Check sheet for the drawn part. Datum: minimum x, y, z corner. Units: mm. Round coordinates to 2 decimals unless told otherwise and drop trailing zeros. Order: outer loops, then holes, each group sorted by start corner. A loop starts at its lowest first (then second) coordinate and runs counter-clockwise, first axis right, second up. Notation, with made-up numbers: M -39,49 L 14,49 A10 cw 14,62 Z; hole C 16.5,-23 d11. An arc over 180 degrees is marked long. Write item = value, one per line. Start each with the question number.
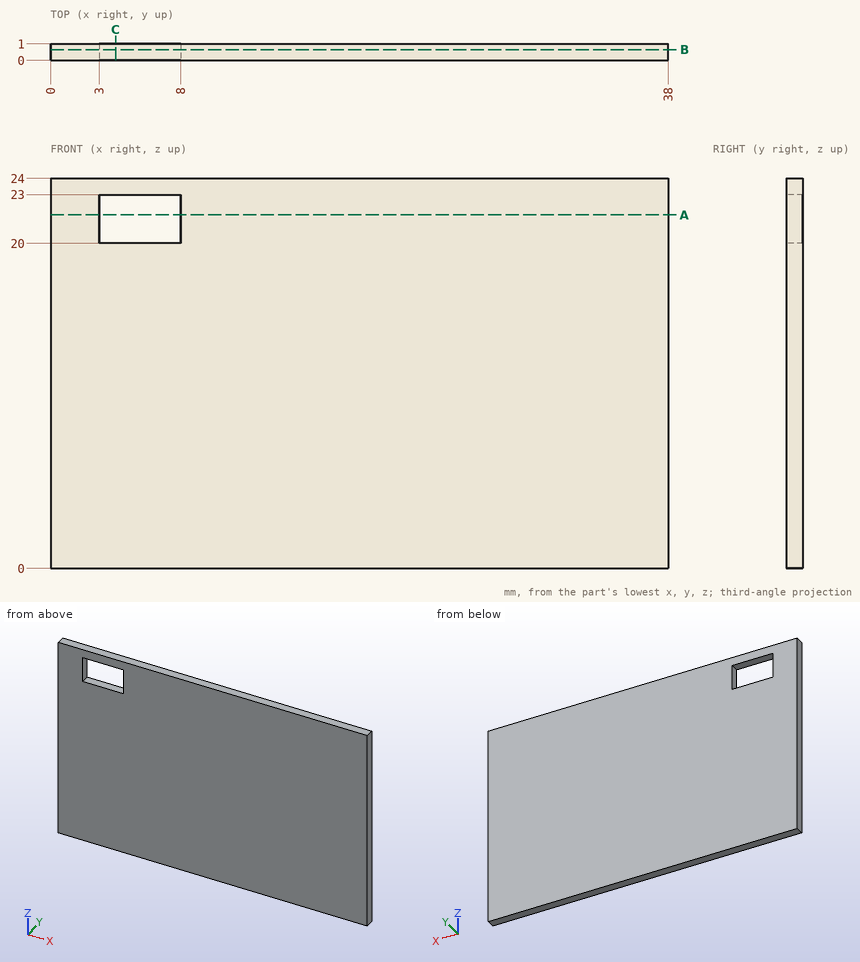
1) Cross-section at A-A, the plane z = 21.75. Enter the section's corners in (x, y).
2) Cross-section at B-B, the plane y = 0.65. Enter the section's corners in (x, z).
3) Cross-section at C-C, the plane x = 4. Enter the section's corners in (y, z), then the cut area to 3 significant figures.
4) Scan lines: probe 1 along X at (y, z) = (0.75, 20.25); probe 2 along Z at (x, y) = (4, 0.3). Record each from-to range of solid material in increasing order.
Geometry results:
q1.outline = M 0,0 L 3,0 L 3,1 L 0,1 Z; M 8,0 L 38,0 L 38,1 L 8,1 Z
q2.outline = M 0,0 L 38,0 L 38,24 L 0,24 Z; hole M 3,20 L 8,20 L 8,23 L 3,23 Z
q3.outline = M 0,0 L 1,0 L 1,20 L 0,20 Z; M 0,23 L 1,23 L 1,24 L 0,24 Z
q3.area = 21.0 mm^2
q4.probe_1 = 0 to 3, 8 to 38
q4.probe_2 = 0 to 20, 23 to 24
